Geometry check sheet. Reference: drawing and pictorial views, mm from the part's lowest x, y, z. A direction names the side the tool comes from. Give positions to 0.01 mm unless a question says otherwise; leave off trailing zeros. Order: outer loops, then holes, each group sorted by start corner. A loop starts at its lowest first (then second) coordinate and runs counter-clockwise, first axis right, second up. Notation, with made-up numbers: M 39.5,76 L 49.5,76 A20 ccw 49.5,112 Z; hole C 11.25,2 d7. An arc over 180 degrees is marked long. Answer as CSV lines item,"result".
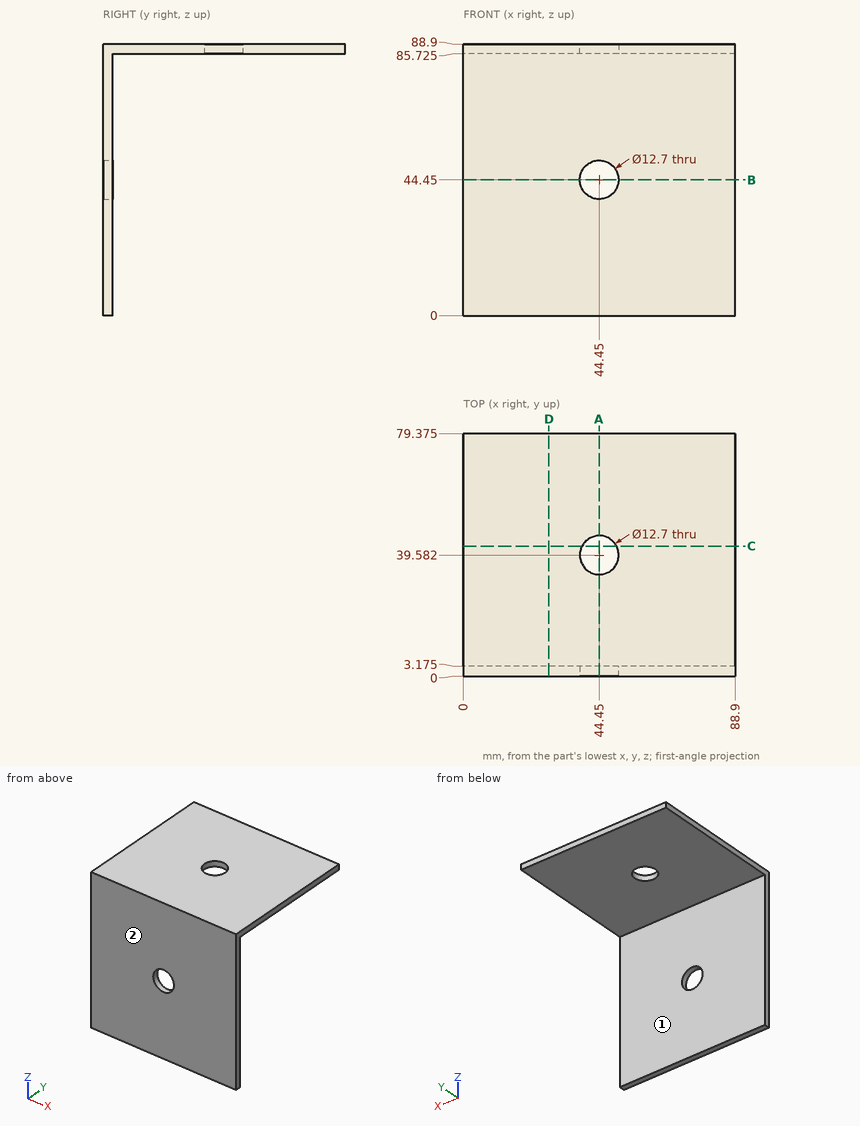
(1) Section check B-B on z = 44.45. Enter the section's corners in (x, y) (1 decimal).
The answers:
outline,"M 0,0 L 38.1,0 L 38.1,3.2 L 0,3.2 Z; M 50.8,0 L 88.9,0 L 88.9,3.2 L 50.8,3.2 Z"
(2) Gauge pin test, flat ends, axial feed: P1, Ø4, axis at x = 36, y = 55, coming from the -Z side (3 decimals); P2, Ø20.5, axis at x = 44.45, z = 44.45, coming from the +Y side (3 decimals). Record the tip position at first contact, or that the pin passes through.
The answers:
P1,"stops at z = 85.725"
P2,"stops at y = 3.175"
(3) Section check D-D on x = 28. Enter the section's corners in (y, z) (1 decimal).
The answers:
outline,"M 0,0 L 3.2,0 L 3.2,85.7 L 79.4,85.7 L 79.4,88.9 L 0,88.9 Z"
(4) Tool access check on the marked faces 1 and 2. Record the directions out of +Z, -Z, +X, -X, +Y, -Y that give a thin tool (end or side, any length) a straight path to the whole face; none if there is none.
The answers:
face 1,"-Z, +X, -X, +Y"
face 2,"+Z, -Z, +X, -X, -Y"
(5) Section check C-C on y = 42.5. Enter the section's corners in (x, z) (1 decimal).
The answers:
outline,"M 0,85.7 L 38.8,85.7 L 38.8,88.9 L 0,88.9 Z; M 50.1,85.7 L 88.9,85.7 L 88.9,88.9 L 50.1,88.9 Z"
(6) Section check A-A on x = 44.45. Enter the section's corners in (y, z) (1 decimal).
The answers:
outline,"M 0,0 L 3.2,0 L 3.2,38.1 L 0,38.1 Z; M 0,50.8 L 3.2,50.8 L 3.2,85.7 L 33.2,85.7 L 33.2,88.9 L 0,88.9 Z; M 45.9,85.7 L 79.4,85.7 L 79.4,88.9 L 45.9,88.9 Z"
(7) Material ranges on line 1 (Z direction, x = 44.45, y = 1.2); line 2 (Y direction, x = 44.45, z = 86.65) (1 decimal); line 3 (Y direction, x = 22.5, z = 45) (1 decimal), recorded low to high.
The answers:
line 1,"z = 0 to 38.1, 50.8 to 88.9"
line 2,"y = 0 to 33.2, 45.9 to 79.4"
line 3,"y = 0 to 3.2"
